Geometry: final body of the model. Coordinates: model frame, mm. A direction names the side the tool comes from. Give positions to 0.01 mm unless a question says otherwise; leave off trailing zeros. Write each loop counter-clockwise with the first axis right and the second up, starting at its lowest first coordinate (ties: lowest second). Pieces come first, ordered by that corner, then holes.
```python
from build123d import *

# Parameters (mm, degrees)
EXTRUDE_1_DEPTH     = 11
CHAMFER_2_SIZE      = 5
CHAMFER_3_SIZE      = 1
SKETCH_2_R          = 2.6
CUT_EXTRUDE_1_DEPTH = 84.385355554
SKETCH_3_R          = 5
CUT_EXTRUDE_2_DEPTH = 5


with BuildPart() as part:
    # Эскиз1 → Бобышка-Вытянуть1 (new body)
    with BuildSketch(Plane.XY):
        Polygon((-5.5, 0.4), (-3.7, 0.4), (-3.7, 0), (3.7, 0), (3.7, 0.4), (10, 0.4), (10, 16.222307726), (-7.950469523, 69.319681931), (-8.350343704, 69.329713846), (-10, 67.370470597), (-48.987732655, 68.348582239), (-50.537069808, 70.388080802), (-50.93694399, 70.398112716), (-51.087422704, 64.4), (-11.227215564, 63.4), (5, 15.4), (5, 5.4), (-5.5, 5.4), align=None)
    extrude(amount=EXTRUDE_1_DEPTH)

    # Фаска2
    chamfer_2_edges = [part.edges().sort_by_distance(p)[0] for p in [
        (5, 5.4, 5.5),
        (-11.227215564, 63.4, 5.5),
    ]]
    chamfer(chamfer_2_edges, length=CHAMFER_2_SIZE)

    # Фаска3
    chamfer_3_edges = [part.edges().sort_by_distance(p)[0] for p in [
        (-51.087422704, 64.4, 5.5),
    ]]
    chamfer(chamfer_3_edges, length=CHAMFER_3_SIZE)

    # Эскиз2 → Вырез-Вытянуть1 (cut, through all)
    with BuildSketch(Plane(origin=(0, 5.4, 0), x_dir=(1, 0, 0), z_dir=(0, 1, 0))):
        with Locations(Location((0, -5.5, 0), (0, 0, 270))):
            Circle(SKETCH_2_R)
    extrude(amount=-CUT_EXTRUDE_1_DEPTH, mode=Mode.SUBTRACT)

    # Эскиз3 → Вырез-Вытянуть2 (cut)
    with BuildSketch(Plane(origin=(0, 5.4, 0), x_dir=(1, 0, 0), z_dir=(0, 1, 0))):
        with Locations((0, -5.5)):
            Circle(SKETCH_3_R)
    extrude(amount=CUT_EXTRUDE_2_DEPTH, mode=Mode.SUBTRACT)


solid = part.part
```
Item 1: Reachability of faces 4 (the face through (-9.164, 68.364, 5.423)), 5 (the face through (7, 0.4, 5)), 6 (the face through (0.78, 2.74, 7.98)) from +Z, -Z, +X, -X, +Y, -Y: full face, straight path, thin tool, end or side. Return the list, or none.
Found:
face 4: +Z, -Z, +Y
face 5: +Z, -Z, +X, -Y
face 6: -Y
Item 2: Line query: L1, parallel to Z at x = 0, y = 2.65; L2, parallel to X at y = 1.1, z = 5.5; L3, parallel to Y at x = -20, z = 9.75. Output: solid intervals per line, ascending.
Found:
L1: z = 0 to 2.9, 8.1 to 11
L2: x = -5.5 to -2.6, 2.6 to 10
L3: y = 63.62 to 67.62
Item 3: Section B-B, the plane z = 2. Return the cut outline in (x, y), plus the area to 3 significant figures.
Found:
outline: (-51.06, 65.4) - (-50.09, 64.37) - (-16.23, 63.53) - (-9.63, 58.66) - (5, 15.4) - (5, 10.4) - (3.57, 8.97) - (3.57, 5.4) - (-5.5, 5.4) - (-5.5, 0.4) - (-3.7, 0.4) - (-3.7, 0) - (3.7, 0) - (3.7, 0.4) - (10, 0.4) - (10, 16.22) - (-7.95, 69.32) - (-8.35, 69.33) - (-10, 67.37) - (-48.99, 68.35) - (-50.54, 70.39) - (-50.94, 70.4) - close
area: 584 mm2
Item 4: Pull-direction query (Z, two-part tool) for faces 1 (the face through (-3, 41, 0)), 2 (the face through (5, 7.3, 5.6)), 3 (the face through (-5, 0.4, 5)); classes: +Z half, -Z half, draft (parallel to the pull), parting line (faces both ways), or undercut.
Found:
face 1: -Z half
face 2: undercut
face 3: draft
Item 5: Pin query (flat end, axial travel): pin 1 Ø5.5 at (y, z) = (14, 4) entering from -X; pin 2 Ø3 at (y, z) = (33, 7.5) entering from -X; pin 3 Ø2 at (x, z) = (-42.5, 9) entering from -Y. Return the tip coordinate at first contact, or that it passes through.
Found:
pin 1: stops at x = 4.54
pin 2: stops at x = -1.46
pin 3: stops at y = 64.16
Item 6: Section D-D, the plane x = -25.5. Return the cut outline in (y, z), plus the area to 3 significant figures.
Found:
outline: (63.76, 0) - (67.76, 0) - (67.76, 11) - (63.76, 11) - close
area: 44.0 mm2
Item 7: Section C-C, the plane y = 41. Return the cut outline in (x, z).
Found:
outline: (-3.65, 0) - (1.62, 0) - (1.62, 11) - (-3.65, 11) - close
Item 8: Section A-A, the plane z = 7. Return the cut outline in (x, y).
Found:
outline: (-51.06, 65.4) - (-50.09, 64.37) - (-16.23, 63.53) - (-9.63, 58.66) - (5, 15.4) - (5, 10.4) - (4.77, 10.17) - (4.77, 5.4) - (2.12, 5.4) - (2.12, 0) - (3.7, 0) - (3.7, 0.4) - (10, 0.4) - (10, 16.22) - (-7.95, 69.32) - (-8.35, 69.33) - (-10, 67.37) - (-48.99, 68.35) - (-50.54, 70.39) - (-50.94, 70.4) - close; (-5.5, 0.4) - (-3.7, 0.4) - (-3.7, 0) - (-2.12, 0) - (-2.12, 5.4) - (-5.5, 5.4) - close
